Model file for the job. Use its own axes, mm. Face numbers are marked on the shaded views. A direction names the side the tool comes from. Give positions to 0.01 mm unless a question says otherwise; leave off trailing zeros. Write each loop counter-clockwise with the first axis right and the second up, starting at its lowest first coordinate (ties: lowest second). Pieces come first, ordered by that corner, then holes. Notation, with made-up numbers: (76.5, 19) - (119.5, 19) arc R26 cw to (119.5, 54) - close; hole circle Ø11 at (79, -15). An arc over 180 degrees is marked (long way). One line per item, written item: value. Start each with the question number.
(1) 3-axis set-ups, long thin cutter, end or side, ignore diameter. For the marked faces 1, 2 and 3: which of +Z, -Z, +X, -X, +Y, -Y reach the whole face in a straight line?
(2) Probe L1, parallel to Y at x = 0, z = 18.5; L2, parallel to X at y = 24, z = 44; L3, parallel to X at y = 24.5, z = 44.45 (3 decimals). List the from-to ranges inside material, lowest first.
(3) Cut at B-B, the plane y = 18.5. List the corners of the cut face in (x, z) (3 decimals).
(4) Drop flat-ended pins along their axis: P1, Ø15, axis at x = 1, z = 46, coming from the +Y side; P2, Ø8, axis at x = -20, y = 48, coming from the +Z side; P3, Ø15, axis at x = 1, z = 42.5, coming from the -Y side; P4, Ø5.5, axis at y = 1, z = 33, coming from the -X side. Give the stop position or say it passes through.
(5) Cut at C-C, the plane z = 38. List the corners of the cut face in (x, y).
(6) Cut at D-D, the plane z = 17.5. List the corners of the cut face in (x, y) (3 decimals), and give its area (3 significant figures).
(7) Mould opens along Y. For the marked faces 4, 5, 6 and 7 say: pulls with the +Y half, pulls with the -Y half, needs draft (parallel to the pull), parting line crosses it, or undercut.
(8) Cut at A-A, the plane x = 0. List the corners of the cut face in (y, z) (3 decimals), and give its area (3 significant figures).
from build123d import *

# Parameters (mm, degrees)
F1_DEPTH  = 25.4
F3_D      = 16.51
F4_W      = 29.644534
F4_H      = 60.19656
F5_DEPTH  = 38.1
F7_DEPTH  = 67.056
F9_D      = 16.51
F11_DEPTH = 41.44285


with BuildPart() as f1:
    # F0 (on Top) → F1 (new body)
    with BuildSketch(Plane.XY):
        with BuildLine():
            Line((26.619583, -49.155481), (26.619583, 49.155481))
            ThreePointArc((26.619583, 49.155481), (0, 75.775065), (-26.619583, 49.155481))
            Line((-26.619583, 49.155481), (-26.619583, -49.155481))
            ThreePointArc((-26.619583, -49.155481), (0, -75.775065), (26.619583, -49.155481))
        make_face()
    extrude(amount=F1_DEPTH)

    # F3 (through all)
    with Locations(Plane.XY.offset(25.4)):
        with Locations((0, 49.155481), (0, -49.155481)):
            Hole(F3_D / 2)

    # F4 (on face) → F5 (join)
    with BuildSketch(Plane.XY.offset(25.4)):
        Rectangle(F4_W, F4_H)
    extrude(amount=F5_DEPTH)

    # F6 (on face) → F7 (cut)
    with BuildSketch(Plane.XZ.offset(30.09828)):
        with BuildLine():
            Line((14.822267, 44.45), (14.822267, 63.5))
            Line((14.822267, 63.5), (-14.822267, 63.5))
            Line((-14.822267, 63.5), (-14.822267, 44.45))
            ThreePointArc((-14.822267, 44.45), (0, 59.272267), (14.822267, 44.45))
        make_face()
    extrude(amount=-F7_DEPTH, mode=Mode.SUBTRACT)

    # F9 (through all)
    with Locations(Plane.XZ.offset(30.09828)):
        with Locations((0, 44.45)):
            Hole(F9_D / 2)

    # F10 (on face) → F11 (cut, through all)
    with BuildSketch(Plane.YZ.offset(14.822267)):
        with BuildLine():
            Line((-13.309792, 65.187737), (-13.309792, 44.45))
            ThreePointArc((-13.309792, 44.45), (0.907487, 27.818035), (15.124765, 44.45))
            Line((15.124765, 44.45), (15.124765, 65.187737))
            Line((15.124765, 65.187737), (-13.309792, 65.187737))
        make_face()
    extrude(amount=-F11_DEPTH, mode=Mode.SUBTRACT)


solid = f1.part
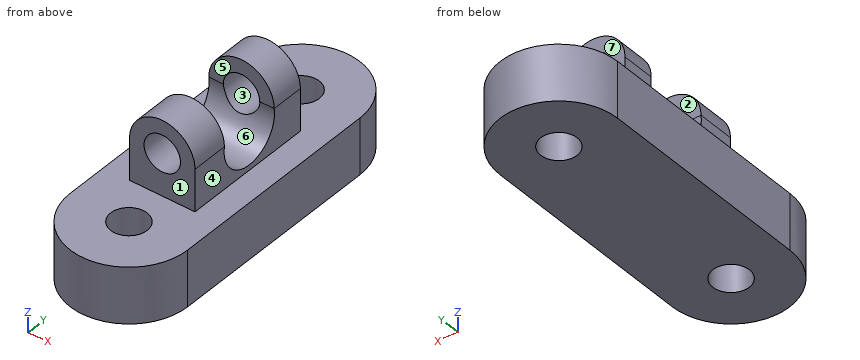
Answers follow:
1. face 1: +Z, +X, -X, -Y
1. face 2: +Z, +X, -X
1. face 3: +Y, -Y
2. L1: y = -75.78 to -57.41, -40.9 to 40.9, 57.41 to 75.78
2. L2: x = -14.82 to -8.24, 8.24 to 14.82
2. L3: x = -14.822 to -8.255, 8.255 to 14.822
3. outline: (-26.62, 0) - (26.62, 0) - (26.62, 25.4) - (14.822, 25.4) - (14.822, 44.45) arc R14.822 ccw to (-14.822, 44.45) - (-14.822, 25.4) - (-26.62, 25.4) - close; hole circle Ø16.51 at (0, 44.45)
4. P1: stops at y = 30.1
4. P2: stops at z = 25.4
4. P3: stops at y = -30.1
4. P4: passes through
5. outline: (-14.82, -30.1) - (-5.15, -30.1) - (-5.15, -12.86) - (-14.82, -12.86) - close; (-14.82, 14.67) - (-5.15, 14.67) - (-5.15, 30.1) - (-14.82, 30.1) - close; (5.15, -30.1) - (14.82, -30.1) - (14.82, -12.86) - (5.15, -12.86) - close; (5.15, 14.67) - (14.82, 14.67) - (14.82, 30.1) - (5.15, 30.1) - close
6. outline: (-26.62, -49.155) arc R26.62 ccw to (26.62, -49.155) - (26.62, 49.155) arc R26.62 ccw to (-26.62, 49.155) - close; hole circle Ø16.51 at (0, -49.155); hole circle Ø16.51 at (0, 49.155)
6. area: 7,030 mm²
7. face 4: needs draft
7. face 5: undercut
7. face 6: undercut
7. face 7: pulls with the +Y half
8. outline: (-75.775, 0) - (-57.41, 0) - (-57.41, 25.4) - (-75.775, 25.4) - close; (-40.9, 0) - (40.9, 0) - (40.9, 25.4) - (30.098, 25.4) - (30.098, 36.195) - (13.983, 36.195) arc R14.393 cw to (-12.168, 36.195) - (-30.098, 36.195) - (-30.098, 25.4) - (-40.9, 25.4) - close; (-30.098, 52.705) - (-13.31, 52.705) - (-13.31, 59.272) - (-30.098, 59.272) - close; (15.125, 52.705) - (30.098, 52.705) - (30.098, 59.272) - (15.125, 59.272) - close; (57.41, 0) - (75.775, 0) - (75.775, 25.4) - (57.41, 25.4) - close
8. area: 3,710 mm²
